Read the model definition and answer for the solid it produces. Units are mm, in the model's axes. Face numbers are marked on the shaded views. Coordinates: 2 decimals unless noted, no trailing zeros. Write each loop counter-clockwise with the first axis right and the second up, starting at its lowest first coordinate (ties: lowest second). Pieces come first, ordered by that corner, then holes. Notation, with made-up numbers: (77.25, -21.5) -> (111.25, -21.5) arc R28 ccw to (111.25, 9.5) -> close; hole circle Ø11 at (46, 4.5). An arc over 180 degrees is marked (long way). Answer as a JSON object with one key per item and string values. Group by question number.
(1) Find section A-A (y = 6). Give the vertices of the cut face in (x, z).
(2) Find section C-C (x = 9). Count the separate pieces of the cut face and the enclosed holes in it, then the cut area to 3 significant figures.
(3) Flat-ended cylindrical pins translate along their axes: P1, Ø3.5, axis at x = 7, z = 1, coming from the -Y side; P2, Ø5, axis at x = 10, y = 17.5, coming from the -Z side; P3, Ø1.4, axis at y = 1, z = -1, coming from the -X side. Find the tip coordinate at first contact, or state that the pin passes through.
(4) Straight lines are drawn through the part: L1, parallel to Z at x = 6.75, y = 5; L2, parallel to Y at x = 0.25, z = -9.75; L3, parallel to Z at x = 13.25, y = 17.5. For each, find the intervals that lie inside material, in ascending order.
(5) Find section B-B (x = -1). Give the vertices of the cut face in (y, z).
(6) Find section D-D (y = 35). Give the vertices of the cut face in (x, z).
(7) For a pull along Z with two mould halves and no side action, classify the marked faces 1, 2 and 3 as +Z half, -Z half, draft (parallel to the pull), parting line (faces both ways), or undercut.
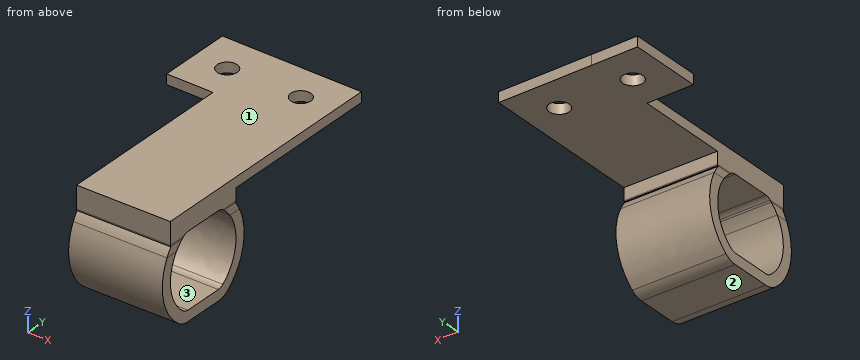
Autodesk Inventor part; units mm, degrees
ref_plane "Work Plane1" through (-71.4012, 38.5222, -12.5) normal (0.0153412, 0.9998823, 0) x (0, 0, 1)
ref_plane "YZ Plane" through (0, 0, 0) normal (1, 0, 0) x (0, 1, 0)
ref_plane "XZ Plane" through (0, 0, 0) normal (0, 1, 0) x (-1, 0, 0)
sketch "Sketch1" plane through (0, 0, 0) normal (0, 0, 1) x (1, 0, 0)
  line L0 (1, 9) -> (14, 9)
  line L1 (1, 3) -> (1, 9)
  line L2 (14, 3) -> (1, 3)
  line L3 (14, 9) -> (14, 3)
  line L4 (1, 12) -> (14, 12)
  line L5 (1, 0) -> (14, 0)
  line L6 (1, 12.5) -> (14, 12.5)
  line L7 (1, -0.5) -> (14, -0.5)
  line L8 (0, 1.4) -> (0, 10.6)
  line L9 (0, -0.5) -> (14, -0.5)
  line L10 (14, -0.5) -> (14, 12.5)
  line L11 (14, 12.5) -> (0, 12.5)
  line L12 (0, 12.5) -> (0, -0.5)
  point P0 (0, 0)
  dimension "d0" = 0.5
  dimension "d1" = 0.5
extrude "Extrusion1" add sketch "Sketch1" along normal blind 2
sketch "Sketch2" plane through (14, -0.5, 0) normal (1, 0, 0) x (0, 0, -1)
  line L0 (10, 9.5) -> (10, 3.5)
  line L1 (10.5, 9.5) -> (10.5, 3.5)
  line L2 (0, 13) -> (0, 0)
  line L3 (0.0028, 13) -> (0, 0)
  arc A0 (5, 0.5) -> (9.8, 2.9) centre (5, 6.5) ccw
  spline S0 degree 3 poles (9.8, 10.1) (9.3822, 10.6561) (8.439, 11.5426) (6.738, 12.3306) (5.0002, 12.5848) (3.2616, 12.3308) (1.5615, 11.5422) (0.6175, 10.6564) (0.2, 10.1) knots 0.000048 0.000048 0.000048 0.000048 1.982593 3.634064 5.285536 6.937008 8.58848 10.571071 10.571071 10.571071 10.571071 weights 1 1 1 1 1 1 1 1 1
  arc A1 (0.2, 2.9) -> (5, 0.5) centre (5, 6.5) ccw
  ellipse E0 centre (0.7683, 3.4229) end of major axis (0.4925, 4.2518) minor radius 0.7558 (0, 3.5) -> (0.2, 2.9) ccw
  ellipse E1 centre (0.7685, 9.5775) end of major axis (1.0457, 10.4061) minor radius 0.7558 (0.2, 10.1) -> (0, 9.5) ccw
  ellipse E2 centre (9.2317, 3.4229) end of major axis (9.5075, 4.2518) minor radius 0.7558 (9.8, 2.9) -> (10, 3.5) ccw
  ellipse E3 centre (9.2318, 9.5768) end of major axis (8.9568, 10.4058) minor radius 0.7558 (10, 9.5) -> (9.7999, 10.1) ccw
  arc A2 (5, 0.0295) -> (10.1758, 2.6168) centre (5, 6.5) ccw
  arc A3 (-0.1717, 2.6115) -> (5, 0.0295) centre (5, 6.5) ccw
  line L4 (10.4705, 3.4977) -> (10.4705, 9.5023)
  ellipse E4 centre (0.7683, 3.4229) end of major axis (0.3339, 4.718) minor radius 1.2242 (-0.4709, 3.5051) -> (-0.1717, 2.6115) ccw
  ellipse E5 centre (0.7685, 9.5775) end of major axis (1.1957, 10.8767) minor radius 1.2233 (-0.1748, 10.3845) -> (-0.4697, 9.4882) ccw
  arc A4 (0.2, 2.9) -> (9.8, 2.9) centre (5, 6.5) ccw
  arc A5 (5, -1.5631) -> (11.4481, 1.6589) centre (5, 6.5) ccw
  arc A6 (-1.4235, 1.6263) -> (5, -1.5631) centre (5, 6.5) ccw
  line L5 (12.0631, 3.4977) -> (12.0631, 9.5023)
  ellipse E6 centre (0.7683, 3.4229) end of major axis (-0.2657, 6.5587) minor radius 2.7801 (-2.0629, 3.5774) -> (-1.4235, 1.6263) ccw
  ellipse E7 centre (0.7685, 9.5775) end of major axis (1.7896, 12.7173) minor radius 2.7798 (-1.4322, 11.3622) -> (-2.0617, 9.4138) ccw
  line L6 (-0.4709, 3.5051) -> (-0.4697, 9.4882)
  line L7 (-2.0629, 3.5774) -> (-2.0617, 9.4138)
  spline S1 degree 5 poles (10.1762, 10.3826) (9.455, 11.3411) (8.5153, 12.1382) (7.3995, 12.6912) (5.0003, 13.2497) (2.6, 12.6917) (1.4857, 12.137) (0.5444, 11.3415) (-0.1764, 10.3824) knots 0 0 0 0 0 0 0.499984 0.499984 0.499984 1 1 1 1 1 1
  spline S2 degree 3 poles (10.1759, 2.6167) (10.3655, 2.8683) (10.4707, 3.1827) (10.4707, 3.4977) knots 0 0 0 0 1 1 1 1
  spline S3 degree 3 poles (10.4707, 9.5023) (10.4707, 9.8173) (10.3655, 10.1318) (10.1757, 10.3833) knots 0 0 0 0 1 1 1 1
  spline S4 degree 4 poles (11.4481, 1.6589) (11.7448, 2.0529) (11.9559, 2.5113) (12.0631, 3.0045) (12.0631, 3.4977) knots 0 0 0 0 0 1 1 1 1 1
  spline S5 degree 4 poles (12.0631, 9.5023) (12.0631, 9.995) (11.9561, 10.4877) (11.7455, 10.9457) (11.4492, 11.3395) knots 0 0 0 0 0 1 1 1 1 1
  spline S6 degree 5 poles (11.4495, 11.3391) (10.5511, 12.5335) (9.3795, 13.5256) (7.9898, 14.2154) (5.0062, 14.9093) (2.0215, 14.2187) (0.6377, 13.5325) (-0.5334, 12.5493) (-1.4322, 11.3622) knots 0 0 0 0 0 0 0.500955 0.500955 0.500955 1 1 1 1 1 1
  point P0 (0, 0.5)
  point P1 (0, 10.6069)
  point P2 (0, 12.8255)
  point P3 (0, 0.1744)
  point P4 (0, 2.393)
  point P5 (0.0005, 2.3924)
  point P6 (0, 0.1743)
  point P7 (0.0027, 12.8276)
  point P8 (0.0023, 10.6096)
extrude "Extrusion2" add sketch "Sketch2" along normal blind 2 contours L3 S6 S5 L5 S4 A5 A6 L2 A3 A2 S2 L4 S3 S1 | S1 E5 L6 E4 A3 L2 A6 E6 L7 E7 S6
sketch "Sketch3" plane through (14, 1.893, 0) normal (1, 0, 0) x (0, 0, -1)
  arc A0 (-0.1717, 0.2185) -> (0, 0) centre (5, 4.107) ccw
  line L0 (0, 0) -> (0, 8.2139)
  arc A1 (0, 8.2139) -> (-0.1748, 7.9915) centre (4.9785, 4.1209) ccw
  ellipse E0 centre (0.7685, 7.1845) end of major axis (0.3413, 5.8853) minor radius 1.2233 (-0.1748, 7.9915) -> (-0.4697, 7.0952) ccw
  line L1 (-0.4697, 7.0952) -> (-0.4709, 1.1121)
  ellipse E1 centre (0.7683, 1.03) end of major axis (1.2028, -0.2651) minor radius 1.2242 (-0.4709, 1.1121) -> (-0.1717, 0.2185) ccw
  point P0 (0, -1.893)
extrude "Extrusion3" cut sketch "Sketch3" against normal through all
sketch "Sketch4" plane through (14, -0.5, 0) normal (-1, 0, 0) x (0, 0, 1)
  line L0 (-10.4705, 9.5023) -> (-10.4705, 3.4977)
  ellipse E0 centre (-9.2512, 9.5832) end of major axis (-8.8307, 10.8511) minor radius 1.2058 (-10.1756, 10.3833) -> (-10.4705, 9.5023) ccw
  spline S0 degree 5 poles (-0.0023, 10.6096) (-0.7281, 11.4914) (-1.6474, 12.2152) (-2.7157, 12.7179) (-5.0579, 13.2362) (-7.3991, 12.6912) (-8.5148, 12.1385) (-9.4545, 11.3415) (-10.1756, 10.3833) knots 0 0 0 0 0 0 0.487709 0.487709 0.487709 1 1 1 1 1 1
  line L1 (-0.0027, 12.8276) -> (-0.0023, 10.6096)
  spline S1 degree 5 poles (-11.4492, 11.3395) (-10.5511, 12.5335) (-9.3795, 13.5256) (-7.9898, 14.2154) (-5.4174, 14.8137) (-2.8441, 14.3827) (-1.8061, 14.0228) (-0.8486, 13.496) (-0.0027, 12.8277) knots 0 0 0 0 0 0 0.581033 0.581033 0.581033 1 1 1 1 1 1
  ellipse E1 centre (-9.2769, 9.5918) end of major axis (-8.3583, 12.3614) minor radius 2.7713 (-11.4492, 11.3395) -> (-12.0631, 9.5023) ccw
  line L2 (-12.0631, 3.4977) -> (-12.0631, 9.5023)
  ellipse E2 centre (-9.2769, 3.4079) end of major axis (-10.1984, 6.1767) minor radius 2.7712 (-12.0631, 3.4977) -> (-11.4481, 1.6589) ccw
  arc A0 (-11.4481, 1.6589) -> (0, 0.1743) centre (-5, 6.5) ccw
  line L3 (-0.0005, 2.3924) -> (0, 0.1743)
  arc A1 (-10.1758, 2.6168) -> (-0.0005, 2.3924) centre (-5, 6.5) ccw
  ellipse E3 centre (-9.2512, 3.4164) end of major axis (-9.673, 4.684) minor radius 1.2058 (-10.4705, 3.4977) -> (-10.1758, 2.6168) ccw
  point P0 (0, 0.5)
extrude "Extrusion4" add sketch "Sketch4" along normal up to surface (14 mm away)
sketch "Sketch5" plane through (0, -0.5, 0) normal (0, -1, 0) x (1, 0, 0)
  line L0 (0, 2) -> (14, 2)
  line L1 (0, 2) -> (14, 2)
  line L2 (14, 2) -> (14, 3.5)
  line L3 (14, 3.5) -> (0, 3.5)
  line L4 (0, 3.5) -> (0, 2)
  point P0 (0, 0)
  dimension "d22" = 1.5
ref_plane "Work Plane1" through (-71.4012, 38.5222, -12.5) normal (0.0153412, 0.9998823, 0) x (0, 0, 1)
extrude "Extrusion5" add sketch "Sketch5" against normal up to surface surface through (-71.4012, 38.5222, -12.5) normal (0.0153412, 0.9998823, 0)
sketch "Sketch6" plane through (0, -0.5, 3.5) normal (0, 0, 1) x (1, 0, 0)
  line L0 (14, 0) -> (14, 37.7119)
  line L1 (14, 37.7119) -> (0, 37.9267)
  line L2 (-54.2389, 27.7576) -> (-67.6625, 27.9635)
  line L3 (14, 37.7119) -> (14, 26.7106)
  line L4 (14, 13) -> (14, 37.7119)
  line L5 (14, 26.7106) -> (-6.9975, 27.0328)
  line L6 (14, 37.7119) -> (-6.9975, 38.034)
  line L7 (-6.9975, 38.034) -> (-6.9975, 27.0328)
  point P0 (0, 0.5)
  point P1 (4.9084, 26.8501)
  dimension "d25" = 21
  dimension "d26" = 21
extrude "Extrusion6" add sketch "Sketch6" against normal blind 1.5
sketch "Sketch7" plane through (0, -0.5, 3.5) normal (0, 0, 1) x (1, 0, 0)
  line L0 (14, 0) -> (14, 37.7119)
  line L1 (14, -3.9463) -> (21.7341, -3.9463)
  line L2 (21.7341, -3.9463) -> (21.7341, 19.3789)
  line L3 (21.7341, 19.3789) -> (14, 19.3789)
  line L4 (14, 19.3789) -> (14, -3.9463)
  point P0 (0, 0.5)
extrude "Extrusion7" cut sketch "Sketch7" against normal blind 15.75
sketch "Sketch8" plane through (14, 10.1069, 0) normal (1, 0, 0) x (0, 0, -1)
  ellipse E0 centre (9.2512, -1.0236) end of major axis (8.8307, 0.2442) minor radius 1.2058 (10.4705, -1.1046) -> (10.1756, -0.2236) ccw
  line L0 (10.4705, -7.1091) -> (10.4705, -1.1046)
  ellipse E1 centre (9.2512, -7.1904) end of major axis (9.673, -5.9229) minor radius 1.2058 (10.1758, -7.9901) -> (10.4705, -7.1091) ccw
  arc A0 (0.0005, -8.2145) -> (10.1758, -7.9901) centre (5, -4.1069) ccw
  line L1 (0, -10.4326) -> (0.0005, -8.2145)
  arc A1 (0, -10.4326) -> (11.4481, -8.948) centre (5, -4.1069) ccw
  ellipse E2 centre (9.2769, -7.199) end of major axis (10.1984, -4.4302) minor radius 2.7712 (11.4481, -8.948) -> (12.0631, -7.1091) ccw
  line L2 (12.0631, -1.1046) -> (12.0631, -7.1091)
  ellipse E3 centre (9.2769, -1.0151) end of major axis (8.3583, 1.7545) minor radius 2.7713 (12.0631, -1.1046) -> (11.4492, 0.7326) ccw
  spline S0 degree 5 poles (0.0027, 2.2208) (0.8486, 2.8891) (1.8061, 3.4159) (2.8441, 3.7759) (5.4174, 4.2068) (7.9898, 3.6085) (9.3795, 2.9188) (10.5511, 1.9266) (11.4492, 0.7326) knots 0 0 0 0 0 0 0.418967 0.418967 0.418967 1 1 1 1 1 1
  line L3 (0.0023, 0.0028) -> (0.0027, 2.2208)
  spline S1 degree 5 poles (10.1756, -0.2236) (9.4545, 0.7346) (8.5148, 1.5316) (7.3991, 2.0844) (5.0579, 2.6294) (2.7157, 2.111) (1.6474, 1.6084) (0.7281, 0.8845) (0.0023, 0.0027) knots 0 0 0 0 0 0 0.512291 0.512291 0.512291 1 1 1 1 1 1
  arc A2 (-0.1717, -7.9954) -> (0, -8.2139) centre (5, -4.1069) ccw
  ellipse E4 centre (0.7683, -7.184) end of major axis (1.2028, -8.479) minor radius 1.2242 (-0.4709, -7.1018) -> (-0.1717, -7.9954) ccw
  ellipse E5 centre (0.7685, -1.0294) end of major axis (0.3413, -2.3286) minor radius 1.2233 (-0.1748, -0.2224) -> (-0.4697, -1.1187) ccw
  arc A3 (0, 0) -> (-0.1748, -0.2224) centre (4.9785, -4.093) ccw
  line L4 (-0.4697, -1.1187) -> (-0.4709, -7.1018)
  line L5 (0, 0) -> (0, 2.3931)
  line L6 (0, 2.3931) -> (-2, 2.3931)
  line L7 (0, -10.6069) -> (0, -8.2139)
  line L8 (0, -10.6069) -> (-3.5, -10.6069)
  line L9 (1.2443, -11.2419) -> (1.2443, -9.3759)
  arc A4 (0.0005, -8.2145) -> (10.1758, -7.9901) centre (5, -4.1069) ccw
  arc A5 (0.0005, -8.2145) -> (1.2443, -9.3759) centre (4.9979, -4.1091) ccw
  line L10 (0, -8.2139) -> (-0.1717, -7.9954)
  ellipse E6 centre (0.7683, -7.184) end of major axis (1.2028, -8.479) minor radius 1.2242 (-0.4709, -7.1018) -> (-0.1717, -7.9954) ccw
  line L11 (-0.1717, -7.9954) -> (-0.1717, -10.6069)
  line L12 (0, -10.6069) -> (-0.1717, -10.6069)
  line L13 (0, -10.6069) -> (0, -10.4326)
  arc A6 (0, -10.4326) -> (1.2443, -11.2419) centre (5, -4.1069) ccw
  line L14 (1.2444, 1.1622) -> (1.2444, 3.0282)
  arc A7 (1.2444, 3.0282) -> (0.0027, 2.2208) centre (4.9892, -4.0883) ccw
  line L15 (0, 2.3931) -> (0, 0)
  line L16 (0.0027, 2.2208) -> (0, 2.3931)
  line L17 (0, 2.3931) -> (-0.1717, 2.3931)
  line L18 (-0.1717, 2.3931) -> (-0.1748, -0.2224)
  line L19 (-0.1748, -0.2224) -> (0.0023, 0.0028)
  line L20 (0.0005, -8.2145) -> (0, -8.2139)
  point P0 (0, -10.1069)
extrude "Extrusion8" add sketch "Sketch8" against normal up to surface (14 mm away) contours S1 L3 S0 L14 | L19 L5 L16 L3 | L9 A1 L1 A0 | A3 L18 L6 L5 | L1 L7 L8 L11 A2
sketch "Sketch9" plane through (0, -0.5, 3.5) normal (0, 0, 1) x (1, 0, 0)
  line L0 (0, 0) -> (0, 26.9254)
  line L1 (14, 0) -> (0, 0)
  line L2 (14, 0) -> (14, 37.7119)
  line L3 (14, 37.7119) -> (-6.9975, 38.034)
  line L4 (-6.9975, 38.034) -> (-6.9975, 27.0328)
  line L5 (-6.9975, 27.0328) -> (0, 26.9254)
  line L6 (-6.9975, 38.034) -> (14, 37.7119)
  line L7 (-6.9975, 38.034) -> (14, 26.7132)
  line L8 (14, 13) -> (14, 37.7119)
  line L9 (14, 37.7119) -> (-6.9975, 27.0328)
  line L10 (-6.9975, 38.034) -> (-6.9975, 27.0328)
  line L11 (-6.9975, 32.3723) -> (14, 32.3723)
  line L12 (-6.9975, 32.3723) -> (0.0025, 32.3723)
  line L13 (14, 32.3723) -> (7, 32.3723)
  line L14 (-6.9975, 32.3723) -> (-1.9975, 32.3723)
  line L15 (14, 32.3723) -> (9, 32.3723)
  circle A0 centre (-1.9975, 32.3723) radius 1.5
  circle A1 centre (9, 32.3723) radius 1.5
  point P0 (0, 0.5)
  dimension "d35" = 5
  dimension "d36" = 5
  dimension "d37" = 3
  dimension "d38" = 3
extrude "Extrusion9" cut sketch "Sketch9" against normal blind 3 contours A0 L11 | L11 A0 | A1 L11 | L11 A1
equation "\"d39\" = d37"
properties part number "leftWheeler_3DPrint"
Results below:
{
 "1": {"outline": "(0, -12.06) -> (14, -12.06) -> (14, -10.47) -> (0, -10.47) -> close; (0, 0.47) -> (14, 0.47) -> (14, 3.5) -> (0, 3.5) -> close"},
 "2": {"separate pieces": "2", "enclosed holes": "1", "area": "128 mm2"},
 "3": {"P1": "stops at y = -0.85", "P2": "stops at z = 2", "P3": "stops at x = 0"},
 "4": {"L1": "z = -12.06 to -10.47, 0.47 to 3.5", "L2": "y = -0.52 to 1.61, 10.39 to 12.52", "L3": "z = 2 to 3.5"},
 "5": {"outline": "(26.44, 2) -> (30.75, 2) -> (30.75, 3.5) -> (26.44, 3.5) -> close; (32.99, 2) -> (37.44, 2) -> (37.44, 3.5) -> (32.99, 3.5) -> close"},
 "6": {"outline": "(-7, 2) -> (14, 2) -> (14, 3.5) -> (-7, 3.5) -> close"},
 "7": {"face 1": "+Z half", "face 2": "-Z half", "face 3": "undercut"}
}
